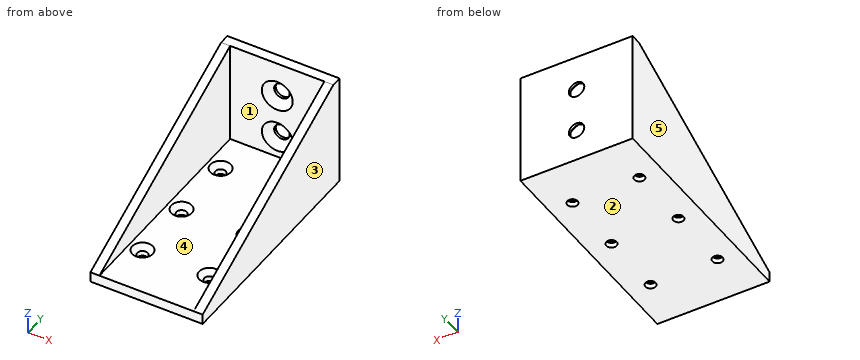
```python
from build123d import *

# Parameters (mm, degrees)
SKETCH_W        = 43.6
SKETCH_H        = 88.5
SKETCH_R        = 2
PAD_DEPTH       = 4
CHAMFER_SIZE    = 2
SKETCH001_W     = 43.6
SKETCH001_H     = 4
PAD001_DEPTH    = 39.85
SKETCH002_R     = 3
HOLE_DEPTH      = 25
HOLE_TIPS_R     = 3
CHAMFER001_SIZE = 3
SKETCH003_W     = 3.5
SKETCH003_H     = 88.5
PAD002_DEPTH    = 39.85
POCKET_DEPTH    = 43.601


with BuildPart() as part:
    # Sketch → Pad (new body)
    with BuildSketch(Plane.XY):
        Rectangle(SKETCH_W, SKETCH_H)
        with Locations((-13, 0)):
            Circle(SKETCH_R, mode=Mode.SUBTRACT)
        with Locations((13, 0)):
            Circle(SKETCH_R, mode=Mode.SUBTRACT)
        with Locations((-13, 25.25)):
            Circle(SKETCH_R, mode=Mode.SUBTRACT)
        with Locations((13, 25.25)):
            Circle(SKETCH_R, mode=Mode.SUBTRACT)
        with Locations((-13, -25.25)):
            Circle(SKETCH_R, mode=Mode.SUBTRACT)
        with Locations((13, -25.25)):
            Circle(SKETCH_R, mode=Mode.SUBTRACT)
    extrude(amount=PAD_DEPTH)

    # Chamfer
    chamfer_edges = [part.edges().sort_by_distance(p)[0] for p in [
        (-15, -25.25, 4),
        (-15, 0, 4),
        (-15, 25.25, 4),
        (11, 25.25, 4),
        (11, 0, 4),
        (11, -25.25, 4),
    ]]
    chamfer(chamfer_edges, length=CHAMFER_SIZE)

    # Sketch001 (on Face4 of Chamfer) → Pad001 (join)
    with BuildSketch(Plane.XY.offset(4)):
        with Locations((0, 42.25)):
            Rectangle(SKETCH001_W, SKETCH001_H)
    extrude(amount=PAD001_DEPTH)

    # Sketch002 (on Face20 of Pad001) → Hole (cut)
    with BuildSketch(Plane(origin=(0, 44.25, 0), x_dir=(-1, 0, 0), z_dir=(0, 1, 0))):
        with Locations((0, 12.55)):
            Circle(SKETCH002_R)
        with Locations((0, 30.05)):
            Circle(SKETCH002_R)
    extrude(amount=-HOLE_DEPTH, mode=Mode.SUBTRACT)

    # Hole tips → Hole tip 1 section 0
    with BuildSketch(Plane(origin=(0, 19.25, 0), x_dir=(-1, 0, 0), z_dir=(0, 1, 0)), mode=Mode.PRIVATE) as hole_tip_1_s0:
        with Locations((0, 12.55)):
            Circle(HOLE_TIPS_R)
    loft([hole_tip_1_s0.sketch, Vertex(0, 17.447418, 12.55)], mode=Mode.SUBTRACT)

    # Hole tips → Hole tip 2 section 0
    with BuildSketch(Plane(origin=(0, 19.25, 0), x_dir=(-1, 0, 0), z_dir=(0, 1, 0)), mode=Mode.PRIVATE) as hole_tip_2_s0:
        with Locations((0, 30.05)):
            Circle(HOLE_TIPS_R)
    loft([hole_tip_2_s0.sketch, Vertex(0, 17.447418, 30.05)], mode=Mode.SUBTRACT)

    # Chamfer001
    chamfer001_edges = [part.edges().sort_by_distance(p)[0] for p in [
        (-3, 40.25, 30.05),
        (-3, 40.25, 12.55),
    ]]
    chamfer(chamfer001_edges, length=CHAMFER001_SIZE)

    # Sketch003 (on Face4 of Chamfer001) → Pad002 (join)
    with BuildSketch(Plane.XY.offset(4)):
        with Locations((-20.05, 0)):
            Rectangle(SKETCH003_W, SKETCH003_H)
        with Locations((20.05, 0)):
            Rectangle(SKETCH003_W, SKETCH003_H)
    extrude(amount=PAD002_DEPTH)

    # Sketch004 (on Face12 of Pad002) → Pocket (cut, through all)
    with BuildSketch(Plane(origin=(-21.8, 0, 0), x_dir=(0, -1, 0), z_dir=(-1, 0, 0))):
        Polygon((-40.254917, 43.850445), (44.398479, 3.93337), (49.801365, 49.127281), (-36.76268, 49.127281), align=None)
    extrude(amount=-POCKET_DEPTH, mode=Mode.SUBTRACT)


solid = part.part
```
Could you check a few things on this model? Use its own coordinates, in mm. Face numbers are marked on the shaded views. A direction names the side the tool comes from. Give positions to 0.01 mm unless a question says otherwise; leave off trailing zeros. Write each loop counter-clockwise with the first axis right and the second up, starting at its lowest first coordinate (ties: lowest second). Pieces come first, ordered by that corner, then holes. Notation, with made-up numbers: (38, 77.25) - (89, 77.25) arc R17 cw to (89, 106.25) - close; hole circle Ø7 at (18, 74.25). An arc over 180 degrees is marked (long way). One line per item, written item: value. Start each with the question number.
Item 1: I'm going to push flat-ended pins straight in: pin 1 (6 mm diameter, centred on y = -25.5, z = 19, fed in from +X); pin 2 (5 mm diameter, centred on x = 5.5, z = 28.5, fed in from -Y); pin 3 (3 mm diameter, centred on x = 1, z = 28, fed in from -Y); pin 4 (6.5 mm diameter, centred on x = 13, y = -25.25, fed in from +Z). Where does each tip first touch, or does it pass through?
Item 2: Please list where these lines run through material, in increasing order: line 1 (X direction, y = 25, z = 1); line 2 (Z direction, x = 0, y = 44.05); line 3 (X direction, y = 12, z = 8). Write a range as from..to.
Item 3: Imagine slicing it at A-A, the plane x = 0. Give the number of separate pieces and of enclosed holes in the cut face, and give its area (3 significant figures).
Item 4: Imagine slicing it at D-D, the plane y = 25.25. List the corners of the cut face in (x, z) for me, and give its area (3 significant figures).
Item 5: If we mould it in two halves opening along X, with no side actions, what happens to the marked faces 3, 4 and 5? For each: +X half, -X half, draft (parallel to the pull), parting line (faces both ways), or undercut.
Item 6: Imagine slicing it at C-C, the plane z = 12.55. List the corners of the cut face in (x, y) for me, and give its area (3 significant figures).
Item 7: Which directions (+Z, -Z, +X, -X, +Y, -Y) give clear straight access to the entire face, cutting with the end or side of a thin tool? Please do the marked faces 1 and 2.
Geometry says:
1. pin 1: through
1. pin 2: y = 40.25
1. pin 3: y = 42.47
1. pin 4: z = 3.25
2. line 1: -21.8..-14.98, -11.02..11.02, 14.98..21.8
2. line 2: 0..9.55, 15.55..27.05, 33.05..43.85
2. line 3: -21.8..-18.3, 18.3..21.8
3. separate pieces: 3
3. enclosed holes: 0
3. area: 447 mm^2
4. outline: (-21.8, 0) - (-15, 0) - (-15, 2) - (-17, 4) - (-18.3, 4) - (-18.3, 36.78) - (-21.8, 36.78) - close; (-11, 0) - (11, 0) - (11, 2) - (9, 4) - (-9, 4) - (-11, 2) - close; (15, 0) - (21.8, 0) - (21.8, 36.78) - (18.3, 36.78) - (18.3, 4) - (17, 4) - (15, 2) - close
4. area: 364 mm^2
5. face 3: +X half
5. face 4: undercut
5. face 5: -X half
6. outline: (-21.8, -26.12) - (-18.3, -26.12) - (-18.3, 40.25) - (-6, 40.25) - (-3, 43.25) - (-3, 44.25) - (-21.8, 44.25) - close; (3, 43.25) - (6, 40.25) - (18.3, 40.25) - (18.3, -26.12) - (21.8, -26.12) - (21.8, 44.25) - (3, 44.25) - close
6. area: 606 mm^2
7. face 1: +Z, -Y
7. face 2: -Z, +X, -X, +Y, -Y
